Check sheet for the modelled part. Datum: model origin and axes. Units: mm. Face numbers are marked on the shaded views. Give positions to 0.01 mm unless a question says otherwise; leave off trailing zeros. Loops run counter-clockwise (first coordinate to the right, second up) from the corner with the lowest first, then second, coordinate; pieces in that order, holes last. Notation, with made-up numbers: M -37,5 L -5,5 A28 cw -5,42 Z; hole C 60.5,3 d4. An arc over 180 degrees is marked long. Use one line per item in the form item = value.
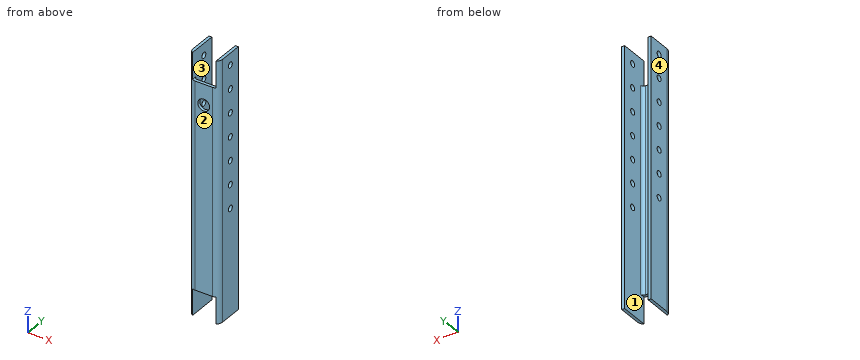
Autodesk Inventor part; units mm, degrees
ref_plane "YZ Plane" through (0, 0, 0) normal (1, 0, 0) x (0, 1, 0)
ref_plane "XZ Plane" through (0, 0, 0) normal (0, 1, 0) x (-1, 0, 0)
ref_plane "XY Plane" through (0, 0, 0) normal (0, 0, 1) x (1, 0, 0)
sketch "Sketch1" plane through (0, 0, 0) normal (0, 0, 1) x (1, 0, 0)
  line L0 (0, 25.4) -> (0, 0)
  line L1 (6.35, -6.35) -> (25.4, -6.35)
  line L2 (31.75, 0) -> (31.75, 25.4)
  line L3 (31.75, 25.4) -> (28.575, 25.4)
  line L4 (28.575, 25.4) -> (28.575, 0)
  line L5 (25.4, -3.175) -> (6.35, -3.175)
  line L6 (3.175, 0) -> (3.175, 25.4)
  line L7 (3.175, 25.4) -> (0, 25.4)
  arc A0 (3.175, 0) -> (6.35, -3.175) centre (6.35, 0) ccw
  arc A1 (0, 0) -> (6.35, -6.35) centre (6.35, 0) ccw
  arc A2 (25.4, -3.175) -> (28.575, 0) centre (25.4, 0) ccw
  arc A3 (25.4, -6.35) -> (31.75, 0) centre (25.4, 0) ccw
  dimension "d0" = 3.175
  dimension "d1" = 25.4
  dimension "d2" = 25.4
  dimension "d3" = 3.175
extrude "Extrusion1" add sketch "Sketch1" along normal blind 279.4
sketch "Sketch2" plane through (31.75, 0, 0) normal (1, 0, 0) x (0, 0, -1)
  line L0 (-279.4, 25.4) -> (-279.4, 0)
  line L1 (0, 25.4) -> (-279.4, 25.4)
  circle A0 centre (-266.7, 12.7) radius 3.175
  dimension "d6" = 6.35
  dimension "d7" = 12.7
  dimension "d8" = 12.7
extrude "Extrusion2" cut sketch "Sketch2" against normal through all
pattern_linear "Rectangular Pattern1" count 7 spacing 25.4 along (0, 0, -1) of "Extrusion2"
sketch "Sketch3" plane through (6.35, -6.35, 0) normal (0, -1, 0) x (1, 0, 0)
  line L0 (19.05, 279.4) -> (0, 279.4)
  circle A0 centre (9.525, 228.6) radius 6.35
  point P0 (-6.35, 0)
  dimension "d14" = 12.7
  dimension "d15" = 50.8
extrude "Extrusion3" cut sketch "Sketch3" against normal up to next
sketch "Sketch4" plane through (6.35, -6.35, 0) normal (0, -1, 0) x (1, 0, 0)
  line L0 (19.05, 279.4) -> (0, 279.4)
  line L1 (0, 0) -> (0, 279.4)
  line L2 (0, 0) -> (19.05, 0)
  line L3 (19.05, 0) -> (19.05, 279.4)
  line L4 (-3.175, 279.4) -> (22.225, 279.4)
  line L5 (22.225, 279.4) -> (22.225, 250.825)
  line L6 (22.225, 250.825) -> (-3.175, 250.825)
  line L7 (-3.175, 250.825) -> (-3.175, 279.4)
  line L8 (-3.175, 165.9576) -> (0, 165.9576) construction
  line L9 (19.05, 165.9576) -> (22.225, 165.9576) construction
  line L10 (-3.175, 0) -> (22.225, 0)
  line L11 (22.225, 0) -> (22.225, 28.575)
  line L12 (22.225, 28.575) -> (-3.175, 28.575)
  line L13 (-3.175, 28.575) -> (-3.175, 0)
  line L14 (-6.35, 279.4) -> (-3.175, 279.4)
  line L15 (-3.175, 279.4) -> (-3.175, 250.825)
  line L16 (-3.175, 250.825) -> (-6.35, 250.825)
  line L17 (-6.35, 250.825) -> (-6.35, 279.4)
  point P0 (-6.35, 0)
  dimension "d18" = 25.4
  dimension "d19" = 28.575
  dimension "d20" = 0
  dimension "d21" = 0
extrude "Extrusion4" cut sketch "Sketch4" against normal through all contours L3 L6 L1 L0 | L4 L5 L6 L3 | L1 L6 L7 L4 | L12 L11 L10 L3 | L3 L2 L1 L12 | L1 L10 L13 L12
properties part number "Frame_OuterConveyorMount" material "Aluminum-6061"
1) Release check for a two-part mould opening along X. For the marked faces 1, 2, 3 and 4 record: pulls with the +X half, pulls with the -X half, needs draft (parallel to the pull), parting line crosses it, or undercut.
Evaluation:
face_1 = undercut
face_2 = needs draft
face_3 = undercut
face_4 = pulls with the -X half
2) Section check B-B (z = 266.7). Record the cut outline in (x, y) (3 decimals), then the cut area to 3 significant figures.
Evaluation:
outline = M 0,0 A6.35 ccw 3.175,-5.499 L 3.175,9.525 L 0,9.525 Z; M 0,15.875 L 3.175,15.875 L 3.175,25.4 L 0,25.4 Z; M 28.575,-5.499 A6.35 ccw 31.75,0 L 31.75,9.525 L 28.575,9.525 Z; M 28.575,15.875 L 31.75,15.875 L 31.75,25.4 L 28.575,25.4 Z
area = 146 mm^2
3) Depth check by flat-ended pin: pin 1 Ø5 at (x, y) = (12, -4) entering from -Z (3 decimals); pin 2 Ø5 at (x, y) = (21.5, -3.5) entering from +Z (3 decimals). Enter the tip coordinate at first touch or a pass-through.
Evaluation:
pin_1 = 28.575
pin_2 = 250.825
4) Section check D-D (x = 14.5). Record the cut outline in (y, z) (3 decimals), then the cut area to 3 significant figures.
Evaluation:
outline = M -6.35,28.575 L -3.175,28.575 L -3.175,222.401 L -6.35,222.401 Z; M -6.35,234.799 L -3.175,234.799 L -3.175,250.825 L -6.35,250.825 Z
area = 666 mm^2
5) Section check C-C (y = 6). Record the cut outline in (x, z) (3 decimals).
Evaluation:
outline = M 0,0 L 3.175,0 L 3.175,279.4 L 0,279.4 Z; M 28.575,0 L 31.75,0 L 31.75,279.4 L 28.575,279.4 Z
6) Scan lines: line 1 (X direction, y = 2, z = 174) (3 decimals); line 2 (Y direction, x = 15, z = 112) (3 decimals); line 3 (X direction, y = -2.5, z = 47.5). Record each from-to range of solid material in increasing order.
Evaluation:
line_1 = 0 to 3.175, 28.575 to 31.75
line_2 = -6.35 to -3.175
line_3 = 0.51 to 4.39, 27.36 to 31.24
7) Section check A-A (z = 215.9). Record the cut outline in (x, y) (3 decimals), then the cut area to 3 significant figures.
Evaluation:
outline = M 0,0 A6.35 ccw 6.35,-6.35 L 25.4,-6.35 A6.35 ccw 31.75,0 L 31.75,9.525 L 28.575,9.525 L 28.575,0 A3.175 cw 25.4,-3.175 L 6.35,-3.175 A3.175 cw 3.175,0 L 3.175,9.525 L 0,9.525 Z; M 0,15.875 L 3.175,15.875 L 3.175,25.4 L 0,25.4 Z; M 28.575,15.875 L 31.75,15.875 L 31.75,25.4 L 28.575,25.4 Z
area = 229 mm^2
